Build history of the part. All positions in model axes, mm. Face numbers are marked on the shaded views. A direction names the side the tool comes from. Round coordinates to 2 decimals unless told otherwise and drop trailing zeros. Write each loop counter-clockwise with the first axis right and the second up, starting at its lowest first coordinate (ties: lowest second). Pieces come first, ordered by that corner, then holes.
1) Flat gauge pins, fed straight in: pin 1 (2.5 mm diameter, centred on x = 0, y = 19.85, fed in from +Z); pin 2 (2 mm diameter, centred on x = -8.5, y = 1, fed in from +Z); pin 3 (1.5 mm diameter, centred on x = 25, y = -25, fed in from -Z). Where does each tip first touch, or does it go through?
2) Which spindle directions (+Z, -Z, +X, -X, +Y, -Y) get a long thin tool onto all of the face, cutting with end or side? Do the marked faces 1 and 2. Say none if no direction does.
3) Saw through at A-A (z = 11.25). Write the cut outline in (x, y), plus the area to 3 significant figures.
4) Pull direction Y, two halves, no side cores. Call the marked faces 3, 4 and 5: +Y half, -Y half, draft (parallel to the pull), parting line (faces both ways), or undercut.
5) Saw through at C-C (x = -20). Write the cut outline in (y, z), plus the area to 3 significant figures.
6) Saw through at D-D (y = -10). Write the cut outline in (x, z) (3 decimals), plus the area to 3 significant figures.
7) Saw through at B-B (y = -1). Write the cut outline in (x, z) (3 decimals).
8) Wall check: probe 1 along Y at (x, z) = (-25, 1.45) (3 decimals); probe 2 along X at (y, z) = (-25, 1.6) (3 decimals); probe 3 along X at (y, z) = (-13, 1.75). Give the ranges that are in metal, low to high.
from build123d import *

# Parameters (mm, degrees)
SKETCH_W         = 65.5
SKETCH_H         = 65.5
PAD_DEPTH        = 10
SKETCH001_R      = 3.55
SKETCH001_R_2    = 2.5
PAD001_DEPTH     = 3
SKETCH002_R      = 2
POCKET_DEPTH     = 8
CHAMFER_SIZE     = 0.2
POCKET001_DEPTH  = 2.5
SKETCH004_W      = 40.5
SKETCH004_H      = 3.5
POCKET002_DEPTH  = 2
SKETCH005_W      = 40.5
SKETCH005_H      = 3.5
POCKET003_DEPTH  = 2
SKETCH006_W      = 65.5
SKETCH006_H      = 7.15
POCKET004_DEPTH  = 4
SKETCH007_W      = 65.5
SKETCH007_H      = 7.15
POCKET005_DEPTH  = 4
SKETCH008_R      = 0.925
POCKET006_DEPTH  = 2.15
CHAMFER001_SIZE2 = 0.25
CHAMFER001_SIZE  = 1
SKETCH009_R      = 5.25
POCKET007_DEPTH  = 1.25
SKETCH010_W      = 8.92708
SKETCH010_H      = 4
POCKET008_DEPTH  = 4
SKETCH011_W      = 8.92708
SKETCH011_H      = 4
POCKET009_DEPTH  = 5


with BuildPart() as part:
    # Sketch → Pad (new body)
    with BuildSketch(Plane.XY):
        Rectangle(SKETCH_W, SKETCH_H)
    extrude(amount=PAD_DEPTH)

    # Sketch001 (on Face6 of Pad) → Pad001 (join)
    with BuildSketch(Plane.XY.offset(10)):
        with Locations((0, 19.85)):
            Circle(SKETCH001_R)
        with Locations((0, -19.85)):
            Circle(SKETCH001_R_2)
    extrude(amount=PAD001_DEPTH)

    # Sketch002 (on Face10 of Pad001) → Pocket (cut)
    with BuildSketch(Plane.XY.offset(13)):
        with Locations((0, 19.85)):
            Circle(SKETCH002_R)
        with Locations((0, -19.85)):
            Circle(SKETCH002_R)
    extrude(amount=-POCKET_DEPTH, mode=Mode.SUBTRACT)

    # Chamfer
    chamfer_edges = [part.edges().sort_by_distance(p)[0] for p in [
        (-3.55, 19.85, 13),
        (-2.5, -19.85, 13),
    ]]
    chamfer(chamfer_edges, length=CHAMFER_SIZE)

    # Sketch003 (on DatumPlane) → Pocket001 (cut)
    with BuildSketch(Plane.XY.offset(5)):
        Polygon((-3.650297, 17.7425), (0, 15.635), (3.650297, 17.7425), (3.650297, 21.9575), (0, 24.065), (-3.650297, 21.9575), align=None)
        Polygon((-3.650297, -21.9575), (0, -24.065), (3.650297, -21.9575), (3.650297, -17.7425), (0, -15.635), (-3.650297, -17.7425), align=None)
    extrude(amount=-POCKET001_DEPTH, mode=Mode.SUBTRACT)

    # Sketch004 (on Face7 of Pocket001) → Pocket002 (cut)
    with BuildSketch(Plane.YZ.offset(32.75)):
        with Locations((0, 5)):
            Rectangle(SKETCH004_W, SKETCH004_H)
    extrude(amount=-POCKET002_DEPTH, mode=Mode.SUBTRACT)

    # Sketch005 (on Face6 of Pocket002) → Pocket003 (cut)
    with BuildSketch(Plane(origin=(-32.75, 0, 0), x_dir=(0, -1, 0), z_dir=(-1, 0, 0))):
        with Locations((0, 5)):
            Rectangle(SKETCH005_W, SKETCH005_H)
    extrude(amount=-POCKET003_DEPTH, mode=Mode.SUBTRACT)

    # Sketch006 (on DatumPlane) → Pocket004 (cut)
    with BuildSketch(Plane.YZ.offset(30.75)):
        with Locations((0, 5)):
            Rectangle(SKETCH006_W, SKETCH006_H)
    extrude(amount=-POCKET004_DEPTH, mode=Mode.SUBTRACT)

    # Sketch007 (on DatumPlane) → Pocket005 (cut)
    with BuildSketch(Plane(origin=(-30.75, 0, 0), x_dir=(0, -1, 0), z_dir=(-1, 0, 0))):
        with Locations((0, 5)):
            Rectangle(SKETCH007_W, SKETCH007_H)
    extrude(amount=-POCKET005_DEPTH, mode=Mode.SUBTRACT)

    # Sketch008 (on Face11 of Pocket005) → Pocket006 (cut)
    with BuildSketch(Plane(origin=(0, 0, 0), x_dir=(1, 0, 0), z_dir=(0, 0, -1))):
        with Locations((-25, 25)):
            Circle(SKETCH008_R)
        with Locations((25, 25)):
            Circle(SKETCH008_R)
        with Locations((-25, -25)):
            Circle(SKETCH008_R)
        with Locations((25, -25)):
            Circle(SKETCH008_R)
    extrude(amount=-POCKET006_DEPTH, mode=Mode.SUBTRACT)

    # Chamfer001
    chamfer001_edges = [part.edges().sort_by_distance(p)[0] for p in [
        (-25.925, -25, 0),
        (24.075, -25, 0),
        (-25.925, 25, 0),
        (24.075, 25, 0),
    ]]
    chamfer001_side = part.faces().sort_by_distance((0, 0, 0))[0]
    chamfer(chamfer001_edges, length=CHAMFER001_SIZE, length2=CHAMFER001_SIZE2, reference=chamfer001_side)

    # Sketch009 (on Face11 of Chamfer001) → Pocket007 (cut)
    with BuildSketch(Plane.XY.offset(10)):
        with Locations((-20, 19.85)):
            Circle(SKETCH009_R)
        with Locations((20, 19.85)):
            Circle(SKETCH009_R)
        with Locations((20, -19.85)):
            Circle(SKETCH009_R)
        with Locations((-20, -19.85)):
            Circle(SKETCH009_R)
    extrude(amount=-POCKET007_DEPTH, mode=Mode.SUBTRACT)

    # Sketch010 (on DatumPlane) → Pocket008 (cut)
    with BuildSketch(Plane(origin=(28, 0, 10), x_dir=(0.939693, 0, -0.34202), z_dir=(0.34202, 0, 0.939693))):
        with Locations((4.46354, 0)):
            Rectangle(SKETCH010_W, SKETCH010_H)
    extrude(amount=POCKET008_DEPTH, mode=Mode.SUBTRACT)

    # Sketch011 (on DatumPlane) → Pocket009 (cut)
    with BuildSketch(Plane(origin=(-28, 0, 10), x_dir=(0.939693, 0, 0.34202), z_dir=(-0.34202, 0, 0.939693))):
        with Locations((-4.46354, 0)):
            Rectangle(SKETCH011_W, SKETCH011_H)
    extrude(amount=POCKET009_DEPTH, mode=Mode.SUBTRACT)


solid = part.part
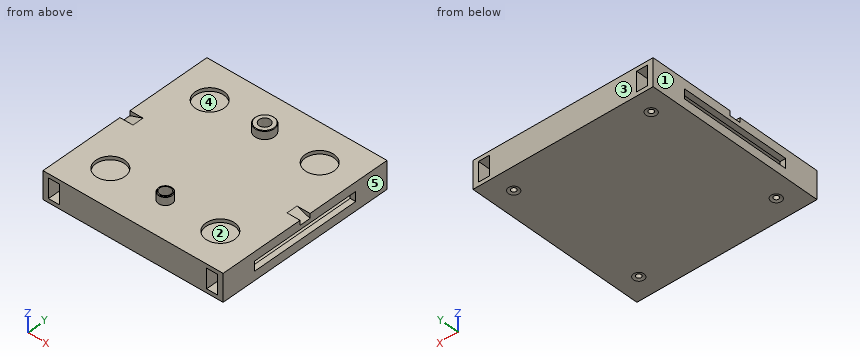
Evaluation:
1. pin 1: stops at z = 2.5
1. pin 2: stops at z = 10
1. pin 3: stops at z = 2.15
2. face 1: +Z, -Z, -X, +Y, -Y
2. face 2: +Z
3. outline: circle Ø7.1 at (0, 19.85); circle Ø5 at (0, -19.85); hole circle Ø4 at (0, -19.85); hole circle Ø4 at (0, 19.85)
3. area: 34.1 mm2
4. face 3: +Y half
4. face 4: undercut
4. face 5: draft
5. outline: (-32.75, 0) - (32.75, 0) - (32.75, 10) - (25.1, 10) - (25.1, 8.75) - (14.6, 8.75) - (14.6, 10) - (-14.6, 10) - (-14.6, 8.75) - (-25.1, 8.75) - (-25.1, 10) - (-32.75, 10) - close
5. area: 629 mm2
6. outline: (-32.75, 0) - (32.75, 0) - (32.75, 3.25) - (30.75, 3.25) - (30.75, 1.425) - (26.75, 1.425) - (26.75, 8.575) - (30.75, 8.575) - (30.75, 6.75) - (32.75, 6.75) - (32.75, 10) - (-32.75, 10) - (-32.75, 6.75) - (-30.75, 6.75) - (-30.75, 8.575) - (-26.75, 8.575) - (-26.75, 1.425) - (-30.75, 1.425) - (-30.75, 3.25) - (-32.75, 3.25) - close
6. area: 584 mm2
7. outline: (-32.75, 0) - (32.75, 0) - (32.75, 3.25) - (30.75, 3.25) - (30.75, 1.425) - (26.75, 1.425) - (26.75, 8.575) - (30.75, 8.575) - (30.75, 6.75) - (32.75, 6.75) - (32.75, 8.271) - (28, 10) - (-28, 10) - (-32.75, 8.271) - (-32.75, 6.75) - (-30.75, 6.75) - (-30.75, 8.575) - (-26.75, 8.575) - (-26.75, 1.425) - (-30.75, 1.425) - (-30.75, 3.25) - (-32.75, 3.25) - close
8. probe 1: y = -32.75 to -25.925, -24.075 to 24.075, 25.925 to 32.75
8. probe 2: x = -32.75 to -30.75, -26.75 to -25.925, -24.075 to 24.075, 25.925 to 26.75, 30.75 to 32.75
8. probe 3: x = -32.75 to -30.75, -26.75 to 26.75, 30.75 to 32.75
